Autodesk Inventor part; units mm, degrees
ref_plane "YZ Plane" through (0, 0, 0) normal (1, 0, 0) x (0, 1, 0)
ref_plane "XZ Plane" through (0, 0, 0) normal (0, 1, 0) x (-1, 0, 0)
ref_plane "XY Plane" through (0, 0, 0) normal (0, 0, 1) x (1, 0, 0)
sketch "Sketch1" plane through (0, 0, 0) normal (0, 1, 0) x (-1, 0, 0)
  circle A0 centre (0, 0) radius 15.875
  circle A1 centre (0, 0) radius 12.7
  dimension "d0" = 31.75
  dimension "d1" = 25.4
extrude "Extrusion1" add sketch "Sketch1" along normal mid plane 355.6
sketch "Sketch2" plane through (0, -177.8, 0) normal (0, -1, 0) x (1, 0, 0)
  circle A0 centre (0, 0) radius 12.7
  circle A1 centre (0, 0) radius 13.4937
  dimension "d4" = 26.9875
extrude "Extrusion2" cut sketch "Sketch2" against normal blind 10
mirror "Mirror1" about plane through (0, 0, 0) normal (0, 1, 0) of "Extrusion2"
properties part number "Acrylic Tube Housing" material "Polycarbonate, Clear"
Geometry check sheet. Reference: the model listing, model coordinates, mm. A direction names the side the tool comes from. Give positions to 0.01 mm unless a question says otherwise; leave off trailing zeros. Loops run counter-clockwise (first coordinate to the right, second up) from the corner with the lowest first, then second, coordinate; pieces in that order, holes last. Notation, with made-up numbers: M 59,-29.75 L 90,-29.75 A15 cw 90,-12.75 Z; hole C -37,29 d10. An arc over 180 degrees is marked long. Write item = value, one per line. Start each with the question number.
1. Thickness scan on probe 1 along Z at (x, y) = (0, 90.5) (3 decimals); probe 2 along Z at (x, y) = (0, 170) (3 decimals); probe 3 along X at (y, z) = (12.5, 3). Record the ranges inside material, lowest first.
2. Section check A-A, the plane x = 0. Enter the section's corners in (y, z) (3 decimals).
3. Go/stop test with flat-tipped pins: P1, Ø10, axis at x = -10.5, y = 58, coming from the +Z side; P2, Ø1.5, axis at x = 5.5, z = 11, coming from the -Y side; P3, Ø3, axis at y = -24.5, z = -8, coming from the +X side; P4, Ø8, axis at x = 6, z = -5.5, coming from the +Y side. Record where each tip stops, or that it passes through.
4. Section check B-B, the plane z = 0. Enter the section's corners in (x, y) (3 decimals).
5. Tool access check on faces 1 (the face through (-2.93, 172.87, 13.17)), 2 (the face through (5, -167.8, -12)), 3 (the face through (7, 177.8, -12)). Record the directions out of +Z, -Z, +X, -X, +Y, -Y that give a thin tool (end or side, any length) a straight path to the whole face; none if there is none.
6. Section check C-C, the plane y = -92.5. Enter the section's corners in (x, z) (3 decimals), plus the area to 3 significant figures.
7. Draft check along X on faces 4 (the face through (2.75, 2.35, -12.4)), 5 (the face through (7, -177.8, -12)), 6 (the face through (3.441, 2.489, -15.497)). Enter one of: +X half, -X half, draft (parallel to the pull), parting line (faces both ways), or undercut.
Values follow:
q1.probe_1 = -15.875 to -12.7, 12.7 to 15.875
q1.probe_2 = -15.875 to -13.494, 13.494 to 15.875
q1.probe_3 = -15.59 to -12.34, 12.34 to 15.59
q2.outline = M -177.8,-15.875 L 177.8,-15.875 L 177.8,-13.494 L 167.8,-13.494 L 167.8,-12.7 L -167.8,-12.7 L -167.8,-13.494 L -177.8,-13.494 Z; M -177.8,13.494 L -167.8,13.494 L -167.8,12.7 L 167.8,12.7 L 167.8,13.494 L 177.8,13.494 L 177.8,15.875 L -177.8,15.875 Z
q3.P1 = 14.89
q3.P2 = -167.8
q3.P3 = 14.48
q3.P4 = through
q4.outline = M -15.875,-177.8 L -13.494,-177.8 L -13.494,-167.8 L -12.7,-167.8 L -12.7,167.8 L -13.494,167.8 L -13.494,177.8 L -15.875,177.8 Z; M 12.7,-167.8 L 13.494,-167.8 L 13.494,-177.8 L 15.875,-177.8 L 15.875,177.8 L 13.494,177.8 L 13.494,167.8 L 12.7,167.8 Z
q5.face_1 = +Y
q5.face_2 = -Y
q5.face_3 = +Z, -Z, +X, -X, +Y
q6.outline = C 0,0 d31.75; hole C 0,0 d25.4
q6.area = 285 mm^2
q7.face_4 = undercut
q7.face_5 = draft
q7.face_6 = parting line
